Read the model definition and answer for the solid it produces. Units are mm, in the model's axes. Give positions to 0.01 mm unless a question says otherwise; leave off trailing zeros. Loops run counter-clockwise (first coordinate to the right, second up) from the corner with the lowest first, then second, coordinate; pieces in that order, holes last. Notation, with made-up numbers: (-19.5, 39) -> (33.5, 39) arc R31 cw to (33.5, 70) -> close; hole circle Ø9 at (27, 63.25). An arc over 180 degrees is marked (long way). Write each question's results on one line, items separated by ' | '. Start each with the question number.
Item 1: Section C-C on y = 863.5 is taken. Write down the section's boundary in (x, z), and give its area (3 significant figures).
Item 2: Section D-D on x = 671.5 is taken. Write down the section's boundary in (y, z).
Item 3: Section A-A on x = 699.5 is taken. Write down the section's boundary in (y, z).
Item 4: Find the intervals of material crossed by line 1 (X direction, y = 868.75, z = 1308); line 2 (X direction, y = 870.25, z = 1306.5); line 3 (Y direction, x = 658.5, z = 1273.5), in increasing order.
Item 5: Section B-B on z = 1298 is taken. Write down the section's boundary in (x, y).
Item 6: Each of these flat-tipped pins is pushed along its axis until it touches: P1, Ø8, axis at x = 686.5, z = 1290, coming from the -Y side; P2, Ø6, axis at x = 668.5, z = 1298, coming from the +Y side. Where does it stop, or does it pass through?
```python
from build123d import *

# Parameters (mm, degrees)
SKETCH1_W             = 50
SKETCH1_H             = 70
BOSS_EXTRUDE1_DEPTH   = 2.54
SKETCH2_W             = 2.15
SKETCH2_H             = 70
BOSS_EXTRUDE2_DEPTH   = 2.54
BOSS_EXTRUDE2_2_DEPTH = 2.54
SKETCH4_W             = 2.15
SKETCH4_H             = 6.68
BOSS_EXTRUDE3_DEPTH   = 70
CUT_EXTRUDE1_DEPTH    = 1123.066858808
SKETCH8_R             = 1.75
BOSS_EXTRUDE4_DEPTH   = 5
FILLET4_R             = 1


with BuildPart() as part:
    # Sketch1 → Boss-Extrude1 (new body)
    with BuildSketch(Plane.XZ.offset(-868.135910235)):
        with Locations((675.180956215, 1301.572260588)):
            Rectangle(SKETCH1_W, SKETCH1_H)
    extrude(amount=BOSS_EXTRUDE1_DEPTH)



with BuildPart() as body_2:
    # Sketch2 → Boss-Extrude2 (new body)
    with BuildSketch(Plane(origin=(0, 869.735910235, 0), x_dir=(1, 0, 0), z_dir=(0, 1, 0))):
        with Locations((651.255956215, -1301.572260588)):
            Rectangle(SKETCH2_W, SKETCH2_H)
    extrude(amount=BOSS_EXTRUDE2_DEPTH)


with BuildPart() as body_3:
    # Sketch2 → Boss-Extrude2 2 (new body)
    with BuildSketch(Plane(origin=(0, 869.735910235, 0), x_dir=(1, 0, 0), z_dir=(0, 1, 0))):
        with Locations((699.105956215, -1301.572260588)):
            Rectangle(SKETCH2_W, SKETCH2_H)
    extrude(amount=BOSS_EXTRUDE2_2_DEPTH)


with BuildPart() as part_1:
    add(part.part)

    add(body_2.part)  # Boss-Extrude3 merges body 2

    add(body_3.part)  # Boss-Extrude3 merges body 3
    # Sketch4 → Boss-Extrude3 (add)
    with BuildSketch(Plane.XY.offset(1336.572260588)):
        with Locations((649.105956215, 868.935910235)):
            Rectangle(SKETCH4_W, SKETCH4_H)
        with Locations((701.255956215, 868.935910235)):
            Rectangle(SKETCH4_W, SKETCH4_H)
    extrude(amount=-BOSS_EXTRUDE3_DEPTH)

    # Sketch6 → Cut-Extrude1 (cut, through all)
    with BuildSketch(Plane(origin=(0, 0, 1266.572260588), x_dir=(-1, 0, 0), z_dir=(0, 0, -1))):
        Polygon((-698.030956215, 869.735910235), (-698.030956215, 868.135910235), (-700.380956215, 868.135910235), (-700.380956215, 869.935910235), (-698.030956215, 869.935910235), align=None)
        Polygon((-652.330956215, 869.935910235), (-652.330956215, 869.735910235), (-652.330956215, 868.135910235), (-649.980956215, 868.135910235), (-649.980956215, 869.935910235), align=None)
    extrude(amount=-CUT_EXTRUDE1_DEPTH, mode=Mode.SUBTRACT)

    # Sketch8 → Boss-Extrude4 (add)
    with BuildSketch(Plane.XZ.offset(-865.595910235)):
        with Locations(Location((651.530956215, 1333.072260588, 0), (0, 0, 180))):
            Circle(SKETCH8_R)
        with Locations(Location((698.830956215, 1333.072260588, 0), (0, 0, 180))):
            Circle(SKETCH8_R)
        with Locations(Location((698.830956215, 1270.072260588, 0), (0, 0, 180))):
            Circle(SKETCH8_R)
        with Locations(Location((651.530956215, 1270.072260588, 0), (0, 0, 180))):
            Circle(SKETCH8_R)
    extrude(amount=BOSS_EXTRUDE4_DEPTH)

    # Fillet4
    fillet4_edges = [part_1.edges().sort_by_distance(p)[0] for p in [
        (702.330956215, 865.595910235, 1301.572260588),
        (702.330956215, 872.275910235, 1301.572260588),
        (648.030956215, 865.595910235, 1301.572260588),
        (648.030956215, 872.275910235, 1301.572260588),
    ]]
    fillet(fillet4_edges, radius=FILLET4_R)


solid = part_1.part
```
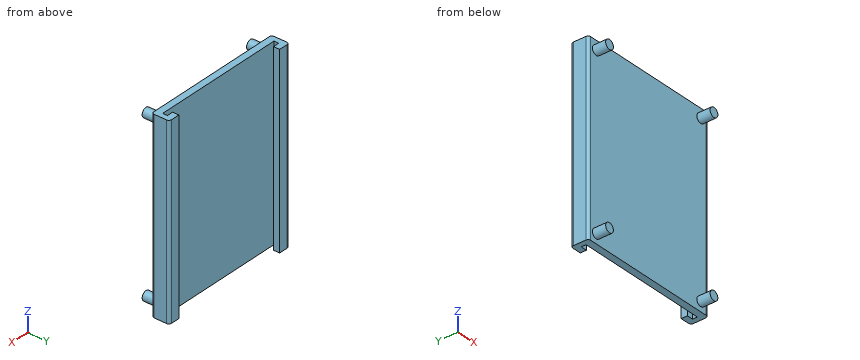
Findings:
1) outline: circle Ø3.5 at (651.53, 1270.07); circle Ø3.5 at (651.53, 1333.07); circle Ø3.5 at (698.83, 1270.07); circle Ø3.5 at (698.83, 1333.07) | area: 38.5 mm2
2) outline: (865.6, 1266.57) -> (868.14, 1266.57) -> (868.14, 1336.57) -> (865.6, 1336.57) -> close
3) outline: (860.6, 1268.46) -> (865.6, 1268.46) -> (865.6, 1266.57) -> (868.14, 1266.57) -> (868.14, 1336.57) -> (865.6, 1336.57) -> (865.6, 1334.69) -> (860.6, 1334.69) -> (860.6, 1331.46) -> (865.6, 1331.46) -> (865.6, 1271.69) -> (860.6, 1271.69) -> close; (869.94, 1266.57) -> (872.28, 1266.57) -> (872.28, 1336.57) -> (869.94, 1336.57) -> close
4) line 1: 648.03 to 649.98, 700.38 to 702.33 | line 2: 648.03 to 652.33, 698.03 to 702.33 | line 3: 865.6 to 868.14
5) outline: (648.03, 866.6) arc R1 ccw to (649.03, 865.6) -> (701.33, 865.6) arc R1 ccw to (702.33, 866.6) -> (702.33, 871.28) arc R1 ccw to (701.33, 872.28) -> (698.03, 872.28) -> (698.03, 869.94) -> (700.38, 869.94) -> (700.38, 868.14) -> (649.98, 868.14) -> (649.98, 869.94) -> (652.33, 869.94) -> (652.33, 872.28) -> (649.03, 872.28) arc R1 ccw to (648.03, 871.28) -> close
6) P1: y = 865.6 | P2: y = 868.14
